```python
from build123d import *

# Parameters (mm, degrees)
SKETCH_1_W           = 38
SKETCH_1_H           = 12
EXTRUDE_4_DEPTH      = 1
SKETCH_2_W           = 31
SKETCH_2_H           = 11.4
EXTRUDE_5_DEPTH      = 3
SKETCH_3_W           = 1.2
SKETCH_3_H           = 1.2
EXTRUDE_6_DEPTH      = 2
EXTRUDE_7_DEPTH      = 2
EXTRUDE_7_DEPTH_BACK = 6
SKETCH_3_5_W         = 1.2
SKETCH_3_5_H         = 1.2


with BuildPart() as part:
    # ｽｹｯﾁ1 → ﾎﾞｽ - 押し出し4 (new body)
    with BuildSketch(Plane.XY):
        Rectangle(SKETCH_1_W, SKETCH_1_H)
    extrude(amount=EXTRUDE_4_DEPTH)

    # ｽｹｯﾁ2 → ﾎﾞｽ - 押し出し5 (add)
    with BuildSketch(Plane.XY):
        with Locations((0.5, 0)):
            Rectangle(SKETCH_2_W, SKETCH_2_H)
    extrude(amount=EXTRUDE_5_DEPTH)

    # ｽｹｯﾁ3 → ﾎﾞｽ - 押し出し6 (add)
    with BuildSketch(Plane.XY):
        with Locations((-17.5, 3.8)):
            Rectangle(SKETCH_3_W, SKETCH_3_H)
        with Locations((-17.5, 1.3)):
            Rectangle(SKETCH_3_W, SKETCH_3_H)
        with Locations((-17.5, -1.2)):
            Rectangle(SKETCH_3_W, SKETCH_3_H)
        with Locations((-17.5, -3.7)):
            Rectangle(SKETCH_3_W, SKETCH_3_H)
    extrude(amount=EXTRUDE_6_DEPTH)

    # ｽｹｯﾁ3<5> → ﾎﾞｽ - 押し出し7 (add, two sides: drawn at the far end of the back side and taken through both)
    with BuildSketch(Plane.XY.offset(-EXTRUDE_7_DEPTH_BACK)):
        with Locations((-17.5, 3.8)):
            Rectangle(SKETCH_3_5_W, SKETCH_3_5_H)
        with Locations((-17.5, 1.3)):
            Rectangle(SKETCH_3_5_W, SKETCH_3_5_H)
        with Locations((-17.5, -1.2)):
            Rectangle(SKETCH_3_5_W, SKETCH_3_5_H)
        with Locations((-17.5, -3.7)):
            Rectangle(SKETCH_3_5_W, SKETCH_3_5_H)
    extrude(amount=EXTRUDE_7_DEPTH + EXTRUDE_7_DEPTH_BACK)


solid = part.part
```
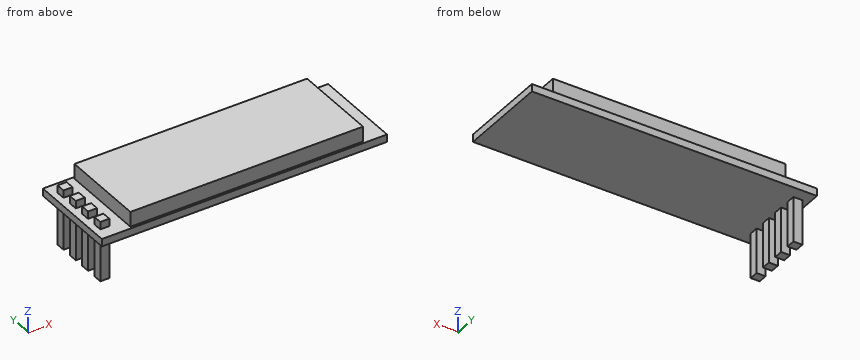
Could you check a few things on this model? Use its own coordinates, in mm. Round coordinates to 2 decimals unless told otherwise and drop trailing zeros. Loops run counter-clockwise (first coordinate to the right, second up) from the corner with the lowest first, then second, coordinate; pieces in that order, holes last. Notation, with made-up numbers: (-35.75, 87) -> (5.25, 87) arc R22 ccw to (5.25, 125) -> close; hole circle Ø3 at (38.25, 23). An arc over 180 degrees is marked (long way). Put each result on its own line as item: value.
Q1. Please list where these lines run through material, in increasing order: line 1 (X direction, y = -1, z = 1.75); line 2 (X direction, y = -3.75, z = -4); line 3 (Z direction, x = 3.5, y = 4.25). Write a range as from..to.
Checks:
line 1: -18.1..-16.9, -15..16
line 2: -18.1..-16.9
line 3: 0..3
Q2. I want a section at C-C on y = 4.75. Write out the boundary of the cut face in (x, z).
Checks:
outline: (-19, 0) -> (19, 0) -> (19, 1) -> (16, 1) -> (16, 3) -> (-15, 3) -> (-15, 1) -> (-19, 1) -> close
Q3. I want a section at B-B on x = 7. Write out the boundary of the cut face in (y, z).
Checks:
outline: (-6, 0) -> (6, 0) -> (6, 1) -> (5.7, 1) -> (5.7, 3) -> (-5.7, 3) -> (-5.7, 1) -> (-6, 1) -> close
Q4. For pin 1 Ø0.6 at (x, y) = (-17.5, -3.5) entering from +Z; pin 2 Ø2 at (y, z) = (-2.5, 2.5) entering from +X; pin 3 Ø0.6 at (x, z) = (-17.5, -3.5) entering from +Y, each with a flat end and sliding along its axis, tell me the tip position at first contact or that it passes through.
Checks:
pin 1: z = 2
pin 2: x = 16
pin 3: y = 4.4
Q5. I want a section at A-A on z = -2.25. Write out the boundary of the cut face in (x, y), and give its area (3 significant figures).
Checks:
outline: (-18.1, -4.3) -> (-16.9, -4.3) -> (-16.9, -3.1) -> (-18.1, -3.1) -> close; (-18.1, -1.8) -> (-16.9, -1.8) -> (-16.9, -0.6) -> (-18.1, -0.6) -> close; (-18.1, 0.7) -> (-16.9, 0.7) -> (-16.9, 1.9) -> (-18.1, 1.9) -> close; (-18.1, 3.2) -> (-16.9, 3.2) -> (-16.9, 4.4) -> (-18.1, 4.4) -> close
area: 5.76 mm2
